from build123d import *

# Parameters (mm, degrees)
F0_W     = 6.3500022411
F0_H     = 6.3500011563
F0_H_2   = 114.2999988437
F0_H_3   = 6.35
F1_DEPTH = 25
F0_W_2   = 6.35
F2_DEPTH = 60
F0_W_3   = 6.3499994576
F3_DEPTH = 35
F4_DEPTH = 7
F0_W_4   = 29.9864560366
F0_W_5   = 59.3868153334
F5_DEPTH = 3


with BuildPart() as f1:
    # F0 (on Top) → F1 (new body)
    with BuildSketch(Plane.XY):
        with Locations((-73.0249988794, -60.3249994218)):
            Rectangle(F0_W, F0_H)
        with Locations((-73.0249988794, 5.782e-07)):
            Rectangle(F0_W, F0_H_2)
        with Locations((-73.0249988794, 60.325)):
            Rectangle(F0_W, F0_H_3)
    extrude(amount=F1_DEPTH)

    # F0 (on Top) → F2 (join)
    with BuildSketch(Plane.XY):
        Polygon((-39.8635417223, -57.1499988437), (-69.8499977589, -57.1499988437), (-69.8499977589, -63.5), (69.85, -63.5), (69.85, -57.1499988437), (51.0366365343, -57.1499988437), (32.2232730687, -57.1499988437), (25.8732736111, -57.1499988437), (-33.5135417223, -57.1499988437), align=None)
        Polygon((69.85, 63.5), (-69.8499977589, 63.5), (-69.8499977589, 57.15), (-39.8635417223, 57.15), (-33.5135417223, 57.15), (25.8732736111, 57.15), (32.2232730687, 57.15), (51.0366365343, 57.15), (69.85, 57.15), align=None)
        with Locations((73.025, 5.782e-07)):
            Rectangle(F0_W_2, F0_H_2)
        with Locations((73.025, -60.3249994218)):
            Rectangle(F0_W_2, F0_H)
        with Locations((73.025, 60.325)):
            Rectangle(F0_W_2, F0_H_3)
    extrude(amount=F2_DEPTH)

    # F0 (on Top) → F3 (join)
    with BuildSketch(Plane.XY):
        with Locations((-36.6885417223, 5.782e-07)):
            Rectangle(F0_W_2, F0_H_2)
        with Locations((29.0482733399, 5.782e-07)):
            Rectangle(F0_W_3, F0_H_2)
    extrude(amount=F3_DEPTH)

    # F0 (on Top) → F4 (join)
    with BuildSketch(Plane.XY):
        with BuildLine():
            Line((51.0366365343, 55.0795492828), (51.0366365343, 57.15))
            Line((51.0366365343, 57.15), (32.2232730687, 57.15))
            Line((32.2232730687, 57.15), (32.2232730687, -57.1499988437))
            Line((32.2232730687, -57.1499988437), (51.0366365343, -57.1499988437))
            Line((51.0366365343, -57.1499988437), (51.0366365343, -55.5998345017))
            ThreePointArc((51.0366365343, -55.5998345017), (38.0366365343, -42.5998345017), (51.0366365343, -29.5998345017))
            Line((51.0366365343, -29.5998345017), (51.0366365343, -26.8984061778))
            ThreePointArc((51.0366365343, -26.8984061778), (38.0366365343, -13.8984061778), (51.0366365343, -0.8984061778))
            Line((51.0366365343, -0.8984061778), (51.0366365343, 1.5994620398))
            ThreePointArc((51.0366365343, 1.5994620398), (38.0366365343, 14.5994620398), (51.0366365343, 27.5994620398))
            Line((51.0366365343, 27.5994620398), (51.0366365343, 29.0795492828))
            ThreePointArc((51.0366365343, 29.0795492828), (38.0366365343, 42.0795492828), (51.0366365343, 55.0795492828))
        make_face()
        with BuildLine():
            Line((69.85, -57.1499988437), (69.85, 57.15))
            Line((69.85, 57.15), (51.0366365343, 57.15))
            Line((51.0366365343, 57.15), (51.0366365343, 55.0795492828))
            ThreePointArc((51.0366365343, 55.0795492828), (60.2290246898, 51.2719374382), (64.0366365343, 42.0795492828))
            ThreePointArc((64.0366365343, 42.0795492828), (60.2290246898, 32.8871611274), (51.0366365343, 29.0795492828))
            Line((51.0366365343, 29.0795492828), (51.0366365343, 27.5994620398))
            ThreePointArc((51.0366365343, 27.5994620398), (60.2290246898, 23.7918501952), (64.0366365343, 14.5994620398))
            ThreePointArc((64.0366365343, 14.5994620398), (60.2290246898, 5.4070738843), (51.0366365343, 1.5994620398))
            Line((51.0366365343, 1.5994620398), (51.0366365343, -0.8984061778))
            ThreePointArc((51.0366365343, -0.8984061778), (60.2290246898, -4.7060180223), (64.0366365343, -13.8984061778))
            ThreePointArc((64.0366365343, -13.8984061778), (60.2290246898, -23.0907943332), (51.0366365343, -26.8984061778))
            Line((51.0366365343, -26.8984061778), (51.0366365343, -29.5998345017))
            ThreePointArc((51.0366365343, -29.5998345017), (60.2290246898, -33.4074463463), (64.0366365343, -42.5998345017))
            ThreePointArc((64.0366365343, -42.5998345017), (60.2290246898, -51.7922226572), (51.0366365343, -55.5998345017))
            Line((51.0366365343, -55.5998345017), (51.0366365343, -57.1499988437))
            Line((51.0366365343, -57.1499988437), (69.85, -57.1499988437))
        make_face()
    extrude(amount=F4_DEPTH)

    # F0 (on Top) → F5 (join)
    with BuildSketch(Plane.XY):
        with Locations((-54.8567697406, 5.782e-07)):
            Rectangle(F0_W_4, F0_H_2)
        with Locations((-3.8201340556, 5.782e-07)):
            Rectangle(F0_W_5, F0_H_2)
        with BuildLine():
            ThreePointArc((51.0366365343, -29.5998345017), (38.0366365343, -42.5998345017), (51.0366365343, -55.5998345017))
            Line((51.0366365343, -55.5998345017), (51.0366365343, -29.5998345017))
        make_face()
        with BuildLine():
            Line((51.0366365343, -29.5998345017), (51.0366365343, -55.5998345017))
            ThreePointArc((51.0366365343, -55.5998345017), (60.2290246898, -51.7922226572), (64.0366365343, -42.5998345017))
            ThreePointArc((64.0366365343, -42.5998345017), (60.2290246898, -33.4074463463), (51.0366365343, -29.5998345017))
        make_face()
        with BuildLine():
            Line((51.0366365343, -0.8984061778), (51.0366365343, -26.8984061778))
            ThreePointArc((51.0366365343, -26.8984061778), (60.2290246898, -23.0907943332), (64.0366365343, -13.8984061778))
            ThreePointArc((64.0366365343, -13.8984061778), (60.2290246898, -4.7060180223), (51.0366365343, -0.8984061778))
        make_face()
        with BuildLine():
            ThreePointArc((51.0366365343, -0.8984061778), (38.0366365343, -13.8984061778), (51.0366365343, -26.8984061778))
            Line((51.0366365343, -26.8984061778), (51.0366365343, -0.8984061778))
        make_face()
        with BuildLine():
            Line((51.0366365343, 1.5994620398), (51.0366365343, 27.5994620398))
            ThreePointArc((51.0366365343, 27.5994620398), (38.0366365343, 14.5994620398), (51.0366365343, 1.5994620398))
        make_face()
        with BuildLine():
            ThreePointArc((64.0366365343, 14.5994620398), (60.2290246898, 23.7918501952), (51.0366365343, 27.5994620398))
            Line((51.0366365343, 27.5994620398), (51.0366365343, 1.5994620398))
            ThreePointArc((51.0366365343, 1.5994620398), (60.2290246898, 5.4070738843), (64.0366365343, 14.5994620398))
        make_face()
        with BuildLine():
            ThreePointArc((64.0366365343, 42.0795492828), (60.2290246898, 51.2719374382), (51.0366365343, 55.0795492828))
            Line((51.0366365343, 55.0795492828), (51.0366365343, 29.0795492828))
            ThreePointArc((51.0366365343, 29.0795492828), (60.2290246898, 32.8871611274), (64.0366365343, 42.0795492828))
        make_face()
        with BuildLine():
            Line((51.0366365343, 29.0795492828), (51.0366365343, 55.0795492828))
            ThreePointArc((51.0366365343, 55.0795492828), (38.0366365343, 42.0795492828), (51.0366365343, 29.0795492828))
        make_face()
    extrude(amount=F5_DEPTH)


solid = f1.part
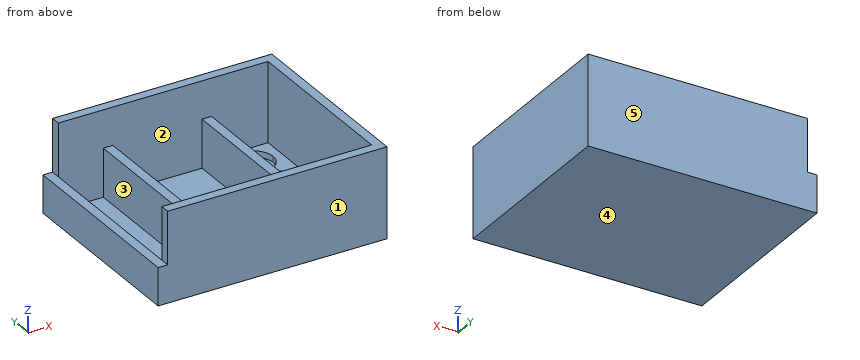
Work out the finished part from the listing and answer in its coordinate system (mm). Face numbers are marked on the shaded views. A direction names the side the tool comes from. Coordinates: 2 decimals unless noted, no trailing zeros. Order: outer loops, then holes, each group sorted by start corner. A loop starts at its lowest first (then second) coordinate and runs counter-clockwise, first axis right, second up. Notation, with made-up numbers: (-19.5, 85.5) - (10.5, 85.5) arc R26 ccw to (10.5, 101.5) - close; hole circle Ø10 at (-2, 22.5). An arc over 180 degrees is marked (long way). Put each result on its own line as item: value. Start each with the question number.
1) Find section D-D (z = 51.5). Give the vertices of the cut face in (x, y).
2) Find section C-C (y = 4). Give the vertices of the cut face in (x, z), plus the area to 3 significant figures.
3) For the marked faces 1 and 2, determine the directions among +Z, -Z, +X, -X, +Y, -Y from which every point of the face is accessible in a straight line to the end or side of a thin tool.
4) For a pull along Y with two mould halves and no side action, classify the marked faces 3, 4 and 5 as released by +Y, released by -Y, zero draft, split by the parting line, or undercut.
5) Find section A-A (x = -14.5). Give the vertices of the cut face in (y, z).
6) Flat-ended cylindrical pins translate along their axes: pin 1 (1.9 mm diameter, centred on x = -38, y = -24, fed in from +Z); pin 2 (3 mm diameter, centred on x = -74, y = 17.5, fed in from +Z); pin 3 (1.5 mm diameter, centred on x = -43.5, y = 27.5, fed in from +Z). Find the tip coordinate at first contact, or state that the pin passes through.
7) Find section B-B (z = 17.5). Give the vertices of the cut face in (x, y).
8) Find the intervals of material crossed by line 1 (X direction, y = -15, z = 33); line 2 (X direction, y = -12.5, z = 20); line 3 (Y direction, x = 12, z = 53), in increasing order. Write a range as from..to.
Results list:
1. outline: (-69.85, -63.5) - (76.2, -63.5) - (76.2, 63.5) - (-69.85, 63.5) - (-69.85, 57.15) - (69.85, 57.15) - (69.85, -57.15) - (-69.85, -57.15) - close
2. outline: (-76.2, 0) - (76.2, 0) - (76.2, 60) - (69.85, 60) - (69.85, 7) - (58.56, 7) - (58.56, 3) - (43.51, 3) - (43.51, 7) - (32.22, 7) - (32.22, 35) - (25.87, 35) - (25.87, 3) - (-33.51, 3) - (-33.51, 35) - (-39.86, 35) - (-39.86, 3) - (-69.85, 3) - (-69.85, 25) - (-76.2, 25) - close
2. area: 1,460 mm^2
3. face 1: +Z, -Z, +X, -X, -Y
3. face 2: +Z
4. face 3: undercut
4. face 4: zero draft
4. face 5: released by +Y
5. outline: (-63.5, 0) - (63.5, 0) - (63.5, 60) - (57.15, 60) - (57.15, 3) - (-57.15, 3) - (-57.15, 60) - (-63.5, 60) - close
6. pin 1: stops at z = 35
6. pin 2: stops at z = 25
6. pin 3: stops at z = 3
7. outline: (-76.2, -63.5) - (76.2, -63.5) - (76.2, 63.5) - (-76.2, 63.5) - close; hole (-69.85, -57.15) - (-39.86, -57.15) - (-39.86, 57.15) - (-69.85, 57.15) - close; hole (-33.51, -57.15) - (25.87, -57.15) - (25.87, 57.15) - (-33.51, 57.15) - close; hole (32.22, -57.15) - (69.85, -57.15) - (69.85, 57.15) - (32.22, 57.15) - close
8. line 1: x = -39.86..-33.51, 25.87..32.22, 69.85..76.2
8. line 2: x = -76.2..-69.85, -39.86..-33.51, 25.87..32.22, 69.85..76.2
8. line 3: y = -63.5..-57.15, 57.15..63.5
